Job drawing, mm, ordinate dimensions from the low corner. One solid piece. A direction names the side the tool comes from. Give positions to 0.01 mm unless a question says otherwise; leave off trailing zeros. Write each loop counter-clockwise with the first axis right and the second up, starting at its lowest first coordinate (ties: lowest second). Pieces come first, ordered by that corner, then holes. Notation, with made-up numbers: (10.5, 54.25) - (19.5, 54.25) arc R10 ccw to (19.5, 64.25) - close; hole circle Ø10 at (42, 7). An arc over 180 degrees is marked (long way). Answer as a JSON object with one key per item and string values.
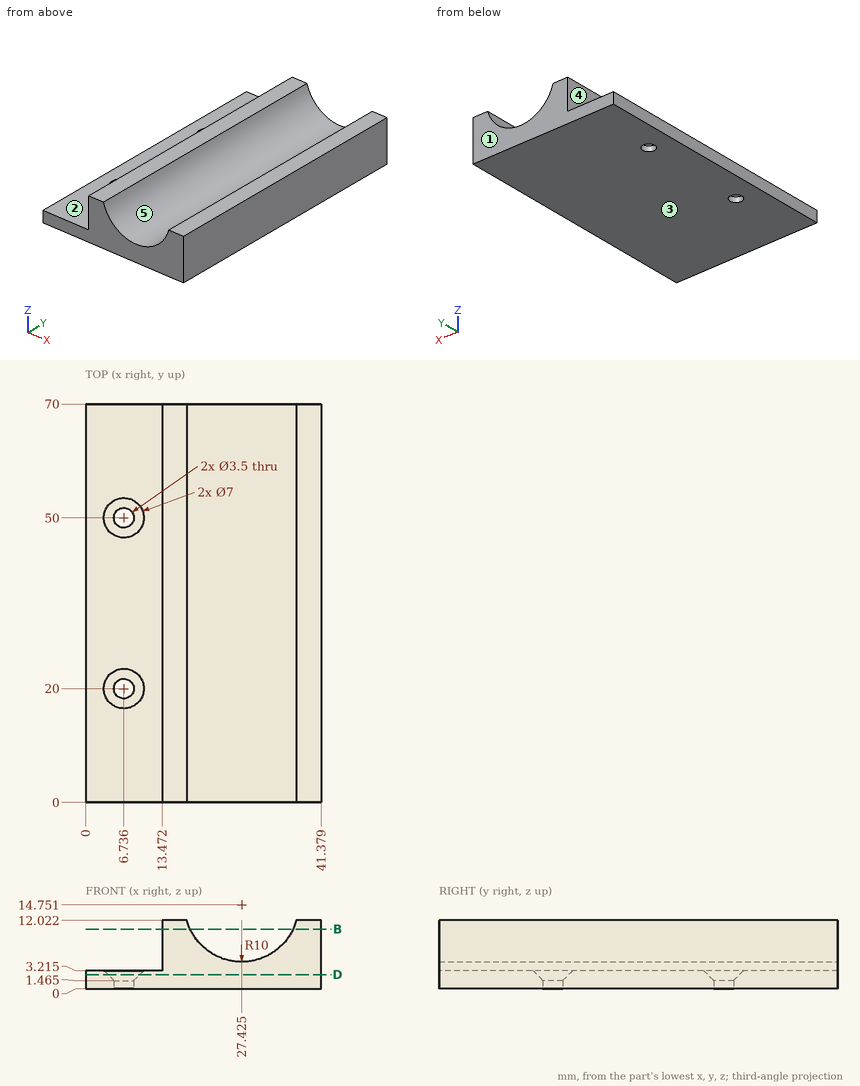
Item 1: Cut at D-D (z = 2.5). Give the cut face in (x, y) (1 decimal), and give its area (3 significant figures).
Entries:
{"outline": "(0, 0) - (41.4, 0) - (41.4, 70) - (0, 70) - close; hole circle Ø5.6 at (6.7, 20); hole circle Ø5.6 at (6.7, 50)", "area": "2,850 mm2"}
Item 2: Mould opens along X. For the marked faces 3, 4 and 5 say: +X half, -X half, draft (parallel to the pull), parting line (faces both ways), or undercut.
Entries:
{"face 3": "draft", "face 4": "-X half", "face 5": "undercut"}
Item 3: Probe line 1 (X direction, y = 50, z = 0.95) (1 decimal); line 2 (Y direction, x = 5.5, z = 1.75) (1 decimal); line 3 (Z direction, x = 5, y = 11.5) (1 decimal). List the from-to ranges inside material, lowest first. Write a range as from..to.
Entries:
{"line 1": "0..5, 8.5..41.4", "line 2": "0..18.4, 21.6..48.4, 51.6..70", "line 3": "0..3.2"}
Item 4: Flat gauge pins, fed straight in: P1, Ø4, axis at x = 6.74, y = 20, coming from the +Z side; P2, Ø2, axis at y = 57.5, z = 6, coming from the -X side; P3, Ø4, axis at x = 11, z = 5.5, coming from the +Y side. Where does each tip first touch, or does it go through?
Entries:
{"P1": "z = 1.72", "P2": "x = 13.47", "P3": "through"}
Item 5: Cut at B-B (z = 10.5). Give the cut face in (x, y).
Entries:
{"outline": "(13.47, 0) - (18.37, 0) - (18.37, 70) - (13.47, 70) - close; (36.48, 0) - (41.38, 0) - (41.38, 70) - (36.48, 70) - close"}
Item 6: Which spindle directions (+Z, -Z, +X, -X, +Y, -Y) get a long thin tool onto all of the face, cutting with end or side? Do the marked faces 1 and 2. Say none if no direction does.
Entries:
{"face 1": "+Z, -Z, +X, -X, +Y", "face 2": "+Z, -X, +Y, -Y"}
